from build123d import *

# Parameters (mm, degrees)
F0_W     = 100
F0_H     = 50
F0_R     = 5
F1_DEPTH = 5
F2_R     = 15
F3_SIZE  = 1
F4_SIZE  = 1


with BuildPart() as f1:
    # F0 (on Top) → F1 (new body)
    with BuildSketch(Plane.XY):
        Rectangle(F0_W, F0_H)
        with Locations((-35, -10)):
            Circle(F0_R, mode=Mode.SUBTRACT)
        with Locations((35, -10)):
            Circle(F0_R, mode=Mode.SUBTRACT)
        with Locations((-20, 10)):
            Circle(F0_R, mode=Mode.SUBTRACT)
        with Locations((20, 10)):
            Circle(F0_R, mode=Mode.SUBTRACT)
    extrude(amount=F1_DEPTH)

    # F2
    f2_edges = [f1.edges().sort_by_distance(p)[0] for p in [
        (-50, 25, 2.5),
        (-50, -25, 2.5),
        (50, -25, 2.5),
        (50, 25, 2.5),
    ]]
    fillet(f2_edges, radius=F2_R)

    # F3
    f3_edges = [f1.edges().sort_by_distance(p)[0] for p in [
        (-25, 10, 5),
        (-40, -10, 5),
        (-25, 10, 0),
        (-40, -10, 0),
        (15, 10, 5),
        (15, 10, 0),
        (30, -10, 5),
        (30, -10, 0),
    ]]
    chamfer(f3_edges, length=F3_SIZE)

    # F4
    f4_edges = [f1.edges().sort_by_distance(p)[0] for p in [
        (-45.606602, 20.606602, 5),
        (-50, 0, 0),
    ]]
    chamfer(f4_edges, length=F4_SIZE)


solid = f1.part
The listing builds one solid part. Answer for the finished solid, in the listing's coordinates (mm). Round coordinates to 2 decimals unless told otherwise and drop trailing zeros. Order: outer loops, then holes, each group sorted by start corner. A loop starts at its lowest first (then second) coordinate and runs counter-clockwise, first axis right, second up. Notation, with made-up numbers: (-10, 84.25) -> (14, 84.25) arc R22 cw to (14, 110.25) -> close; hole circle Ø1 at (-25.75, -5). An arc over 180 degrees is marked (long way). One line per item, written item: value.
Item 1: Given P1, Ø11.5, axis at x = -20, y = 10, coming from the -Z side; P2, Ø11.5, axis at x = 20, y = 10, coming from the +Z side; P3, Ø8, axis at x = -35, y = -10, coming from the -Z side; P4, Ø3, axis at y = -17.5, z = 1, coming from the -X side, each flat-ended and moving along its own axis, determine where each tip first touches the part or whether it passes through.
Taken from the geometry:
P1: stops at z = 0.25
P2: stops at z = 4.75
P3: passes through
P4: stops at x = -48.75
Item 2: Find section B-B, the plane x = -20. Give the vertices of the cut face in (y, z).
Taken from the geometry:
outline: (-25, 1) -> (-24, 0) -> (4, 0) -> (5, 1) -> (5, 4) -> (4, 5) -> (-24, 5) -> (-25, 4) -> close; (15, 1) -> (16, 0) -> (24, 0) -> (25, 1) -> (25, 4) -> (24, 5) -> (16, 5) -> (15, 4) -> close
Item 3: Find section A-A, the plane z = 2.35. Give the vertices of the cut face in (x, y), then the cut area to 3 significant figures.
Taken from the geometry:
outline: (-50, -10) arc R15 ccw to (-35, -25) -> (35, -25) arc R15 ccw to (50, -10) -> (50, 10) arc R15 ccw to (35, 25) -> (-35, 25) arc R15 ccw to (-50, 10) -> close; hole circle Ø10 at (-35, -10); hole circle Ø10 at (-20, 10); hole circle Ø10 at (20, 10); hole circle Ø10 at (35, -10)
area: 4,490 mm2
Item 4: Straight lines are drawn through the part: L1, parallel to Y at x = -20, z = 2.95; L2, parallel to X at y = 6, z = 4.1; L3, parallel to Y at x = 35, z = 2. For each, find the intervals that lie inside material, in ascending order.
Taken from the geometry:
L1: y = -25 to 5, 15 to 25
L2: x = -49.9 to -23.16, -16.84 to 16.84, 23.16 to 49.9
L3: y = -25 to -15, -5 to 25
